Here's how the part is built. I have some questions about the finished solid (model axes, mm). Give positions to 0.01 mm unless a question says otherwise; leave off trailing zeros. Loops run counter-clockwise (first coordinate to the right, second up) from the corner with the lowest first, then second, coordinate; pieces in that order, holes last. Notation, with made-up numbers: (23, -16) - (32, -16) arc R21 cw to (32, 0) - close; hole circle Ø6 at (28, 55). An arc over 180 degrees is marked (long way). Use one line per item in the form item = value.
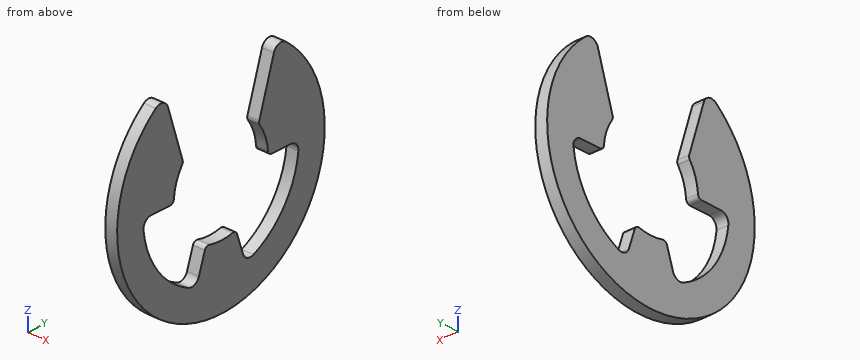
from build123d import *

# Parameters (mm, degrees)
BOSS_EXTRUDE1_DEPTH      = 0.4445
BOSS_EXTRUDE1_DEPTH_BACK = 0.4445
FILLET1_R                = 0.6223
FILLET2_R                = 0.31115


with BuildPart() as part:
    # Sketch3 → Boss-Extrude1 (new, two sides: drawn at the far end of the back side and taken through both)
    with BuildSketch(Plane(origin=(0, 0, 0), x_dir=(0, 0, -1), z_dir=(1, 0, 0)).offset(-BOSS_EXTRUDE1_DEPTH_BACK)):
        with BuildLine():
            Line((3.614483366, -1.204827789), (5.969727365, -1.989909122))
            ThreePointArc((5.969727365, -1.989909122), (3.679374344, -5.104859211), (0, -6.292645161))
            Line((0, -6.292645161), (0, -3.81))
            ThreePointArc((0, -3.81), (-1.204827789, -3.614483366), (-2.286, -3.048))
            Line((-2.286, -3.048), (-7.048739855, -4.535767901))
            ThreePointArc((-7.048739855, -4.535767901), (8.382, 0), (-7.048739855, 4.535767901))
            Line((-7.048739855, 4.535767901), (-2.286, 3.048))
            ThreePointArc((-2.286, 3.048), (-1.204827789, 3.614483366), (0, 3.81))
            Line((0, 3.81), (0, 6.292645161))
            ThreePointArc((0, 6.292645161), (3.679374344, 5.104859211), (5.969727365, 1.989909122))
            Line((5.969727365, 1.989909122), (3.614483366, 1.204827789))
            ThreePointArc((3.614483366, 1.204827789), (3.81, 0), (3.614483366, -1.204827789))
        make_face()
    extrude(amount=BOSS_EXTRUDE1_DEPTH + BOSS_EXTRUDE1_DEPTH_BACK)

    # Fillet1
    fillet1_edges = [part.edges().sort_by_distance(p)[0] for p in [
        (0, 1.989909122, -5.969727365),
        (0, 6.292645161, 0),
        (0, 4.535767901, 7.048739855),
        (0, -4.535767901, 7.048739855),
        (0, -6.292645161, 0),
        (0, -1.989909122, -5.969727365),
    ]]
    fillet(fillet1_edges, radius=FILLET1_R)

    # Fillet2
    fillet2_edges = [part.edges().sort_by_distance(p)[0] for p in [
        (0, 1.204827789, -3.614483366),
        (0, 3.81, 0),
        (0, 3.048, 2.286),
        (0, -3.048, 2.286),
        (0, -3.81, 0),
        (0, -1.204827789, -3.614483366),
    ]]
    fillet(fillet2_edges, radius=FILLET2_R)


solid = part.part
(1) If I drill on probe 1 along Y at (x, z) = (-0.25, -4.75); probe 2 along Y at (x, z) = (0.1, 4); probe 3 along Y at (x, z) = (0.3, -2.25), over which ranges is the centre line in solid material (lowest first)?
Geometry says:
probe_1 = -6.91 to -4.13, -1.58 to 1.58, 4.13 to 6.91
probe_2 = -7.37 to -3.58, 3.58 to 7.37
probe_3 = -8.07 to -5.88, 5.88 to 8.07
(2) If we section it at B-B (x = -0.2): List the corners of the cut face in (y, z) for me, plus the area to 3 significant figures.
Geometry says:
outline = (-6.25, -0.69) arc R0.62 cw to (-5.64, 0) - (-4.11, 0) arc R0.31 ccw to (-3.8, 0.29) arc R3.81 cw to (-3.14, 2.16) arc R0.31 ccw to (-3.09, 2.43) - (-4.28, 6.22) arc R0.62 ccw to (-5.26, 6.52) arc R8.38 ccw (long way) to (5.26, 6.52) arc R0.62 ccw to (4.28, 6.22) - (3.09, 2.43) arc R0.31 ccw to (3.14, 2.16) arc R3.81 cw to (3.8, 0.29) arc R0.31 ccw to (4.11, 0) - (5.64, 0) arc R0.62 cw to (6.25, -0.69) arc R6.29 cw to (2.63, -5.72) arc R0.62 cw to (1.78, -5.35) - (1.3, -3.9) arc R0.31 ccw to (0.93, -3.7) arc R3.81 cw to (-0.93, -3.7) arc R0.31 ccw to (-1.3, -3.9) - (-1.78, -5.35) arc R0.62 cw to (-2.63, -5.72) arc R6.29 cw to start
area = 106 mm²
(3) If we section it at A-A (z = 1.5): List the corners of the cut face in (x, y) for me, plus the area to 3 significant figures.
Geometry says:
outline = (-0.44, -8.25) - (0.44, -8.25) - (0.44, -3.5) - (-0.44, -3.5) - close; (-0.44, 3.5) - (0.44, 3.5) - (0.44, 8.25) - (-0.44, 8.25) - close
area = 8.44 mm²
(4) For P1, Ø2, axis at y = 1.5, z = 4, coming from the -X side, with a flat end and sliding along its axis, tell me the tip position at first contact or that it passes through.
Geometry says:
P1 = through
(5) If we section it at C-C (y = -6): List the corners of the cut face in (x, z) for me, plus the area to 4 significant figures.
Geometry says:
outline = (-0.44, -5.85) - (0.44, -5.85) - (0.44, -1.9) - (-0.44, -1.9) - close; (-0.44, -0.12) - (0.44, -0.12) - (0.44, 5.85) - (-0.44, 5.85) - close
area = 8.825 mm²
(6) If we section it at D-D (y = 0): List the corners of the cut face in (x, z) for me, plus the area to 3 significant figures.
Geometry says:
outline = (-0.44, -8.38) - (0.44, -8.38) - (0.44, -3.81) - (-0.44, -3.81) - close
area = 4.06 mm²
